```python
from build123d import *

# Parameters (mm, degrees)
SKETCH2_R                        = 25.4
SKETCH2_R_2                      = 14.2875
BOSS_EXTRUDE1_DEPTH              = 38.1
CUT_EXTRUDE1_REACH               = 54.363
SKETCH3_W                        = 25.4
SKETCH3_H                        = 1.5875
CUT_EXTRUDE2_REACH               = 54.363
SKETCH4_R                        = 3.0226
TAP_DRILL_FOR_M4X0_7_TAP1_REACH  = 61.824
TAP_DRILL_FOR_M4X0_7_TAP1_BORE_R = 1.65
CUT_EXTRUDE5_REACH               = 70.392
CUT_EXTRUDE5_END_RADIUS          = 3.0226
SKETCH11_R                       = 1.65
CUT_EXTRUDE6_REACH               = 54.363
TAP_DRILL_FOR_M3X0_5_TAP2_D      = 2.5
TAP_DRILL_FOR_M3X0_5_TAP2_DEPTH  = 4.572
TAP_DRILL_FOR_M3X0_5_TAP2_TIP    = 0.751075774
TAP_DRILL_FOR_M5X0_8_TAP1_REACH  = 55.583
TAP_DRILL_FOR_M5X0_8_TAP1_BORE_R = 2.1
SKETCH15_R                       = 2.665
CUT_EXTRUDE7_DEPTH               = 53.7470617
CUT_EXTRUDE8_REACH               = 59.143
SKETCH19_R                       = 5


with BuildPart() as part:
    # Sketch2 → Boss-Extrude1 (new body)
    with BuildSketch(Plane(origin=(0, 0, 0), x_dir=(1, 0, 0), z_dir=(0, 1, 0))):
        with Locations(Location((0, 0, 0), (0, 0, 90))):
            Circle(SKETCH2_R)
        with Locations(Location((0, 0, 0), (0, 0, 90))):
            Circle(SKETCH2_R_2, mode=Mode.SUBTRACT)
    extrude(amount=BOSS_EXTRUDE1_DEPTH)

    # Sketch3 → Cut-Extrude1 (cut, up to next)
    with BuildSketch(Plane(origin=(0, 38.1, 0), x_dir=(1, 0, 0), z_dir=(0, 1, 0)), mode=Mode.PRIVATE) as cut_extrude1_sk1:
        with Locations((-12.7, 0)):
            Rectangle(SKETCH3_W, SKETCH3_H)
    cut_extrude1_tool1 = extrude(cut_extrude1_sk1.sketch, amount=-CUT_EXTRUDE1_REACH, mode=Mode.PRIVATE) & part.part
    add(cut_extrude1_tool1.solids().sort_by_distance((-12.7, 38.1, 0))[0], mode=Mode.SUBTRACT)

    # Sketch4 → Cut-Extrude2 (cut, up to next)
    with BuildSketch(Plane(origin=(0, 38.1, 0), x_dir=(1, 0, 0), z_dir=(0, 1, 0)), mode=Mode.PRIVATE) as cut_extrude2_sk1:
        with Locations(Location((0, -19.84375, 0), (0, 0, 270))):
            Circle(SKETCH4_R)
    cut_extrude2_tool1 = extrude(cut_extrude2_sk1.sketch, amount=-CUT_EXTRUDE2_REACH, mode=Mode.PRIVATE) & part.part
    cut_extrude2 = cut_extrude2_tool1.solids().sort_by_distance((0, 38.1, 19.84375))[0]
    add(cut_extrude2, mode=Mode.SUBTRACT)

    # Tap Drill for M4x0.7 Tap1 bore (on position points) → Tap Drill for M4x0.7 Tap1 (cut, up to next)
    with BuildSketch(Plane(origin=(-19.826514488, 29.109235595, 0.79375), x_dir=(-1, 0, 0), z_dir=(0, 0, -1)), mode=Mode.PRIVATE) as tap_drill_for_m4x0_7_tap1_sk1:
        Circle(TAP_DRILL_FOR_M4X0_7_TAP1_BORE_R)
    tap_drill_for_m4x0_7_tap1_tool1 = extrude(tap_drill_for_m4x0_7_tap1_sk1.sketch, amount=-TAP_DRILL_FOR_M4X0_7_TAP1_REACH, mode=Mode.PRIVATE) & part.part
    # Tap Drill for M4x0.7 Tap1 bore (on position points) → Tap Drill for M4x0.7 Tap1 (cut, up to next)
    with BuildSketch(Plane(origin=(-19.826514488, 29.109235595, 0.79375), x_dir=(-1, 0, 0), z_dir=(0, 0, -1)), mode=Mode.PRIVATE) as tap_drill_for_m4x0_7_tap1_sk2:
        with Locations((0, -20.205281104)):
            Circle(TAP_DRILL_FOR_M4X0_7_TAP1_BORE_R)
    tap_drill_for_m4x0_7_tap1_tool2 = extrude(tap_drill_for_m4x0_7_tap1_sk2.sketch, amount=-TAP_DRILL_FOR_M4X0_7_TAP1_REACH, mode=Mode.PRIVATE) & part.part
    add(tap_drill_for_m4x0_7_tap1_tool1.solids().sort_by_distance((-19.826514, 29.109236, 0.79375))[0], mode=Mode.SUBTRACT)
    add(tap_drill_for_m4x0_7_tap1_tool2.solids().sort_by_distance((-19.826514, 8.903954, 0.79375))[0], mode=Mode.SUBTRACT)

    # Cut-Extrude5: up to this cylinder (the profile starts outside it)
    cut_extrude5_end = Plane(origin=(0, 19.05, 19.84375), z_dir=(0, 1, 0)) * Cylinder(CUT_EXTRUDE5_END_RADIUS, 147.8292, mode=Mode.PRIVATE)
    # Sketch11 → Cut-Extrude5 (cut, up to the surface)
    with BuildSketch(Plane.XY.offset(25.4), mode=Mode.PRIVATE) as cut_extrude5_sk1:
        with Locations((0.006202687, 19.05)):
            Circle(SKETCH11_R)
    cut_extrude5_tool1 = extrude(cut_extrude5_sk1.sketch, amount=-CUT_EXTRUDE5_REACH, mode=Mode.PRIVATE) - cut_extrude5_end
    cut_extrude5 = cut_extrude5_tool1.solids().sort_by_distance((0.006203, 19.05, 25.4))[0]
    add(cut_extrude5, mode=Mode.SUBTRACT)

    # Mirror1: Cut-Extrude2, Cut-Extrude5 across plane
    add(cut_extrude2.mirror(Plane.XY), mode=Mode.SUBTRACT)
    add(cut_extrude5.mirror(Plane.XY), mode=Mode.SUBTRACT)

    # Sketch12 → Cut-Extrude6 (cut, up to next)
    with BuildSketch(Plane(origin=(0, 38.1, 0), x_dir=(1, 0, 0), z_dir=(0, 1, 0)), mode=Mode.PRIVATE) as cut_extrude6_sk1:
        with BuildLine():
            Line((22.86, 11.071603317), (22.86, -11.071603317))
            ThreePointArc((22.86, -11.071603317), (25.4, 0), (22.86, 11.071603317))
        make_face()
    cut_extrude6_tool1 = extrude(cut_extrude6_sk1.sketch, amount=-CUT_EXTRUDE6_REACH, mode=Mode.PRIVATE) & part.part
    add(cut_extrude6_tool1.solids().sort_by_distance((23.880484, 38.1, 0))[0], mode=Mode.SUBTRACT)

    # Tap Drill for M3x0.5 Tap2
    with Locations(Plane(origin=(22.86, 19.05, 0), x_dir=(0, 0, 1), z_dir=(1, 0, 0))):
        with Locations((0, 0)):
            Hole(TAP_DRILL_FOR_M3X0_5_TAP2_D / 2, depth=TAP_DRILL_FOR_M3X0_5_TAP2_DEPTH)
            with Locations((0, 0, -(TAP_DRILL_FOR_M3X0_5_TAP2_DEPTH + TAP_DRILL_FOR_M3X0_5_TAP2_TIP / 2))):  # 118° drill point
                Cone(0, TAP_DRILL_FOR_M3X0_5_TAP2_D / 2, TAP_DRILL_FOR_M3X0_5_TAP2_TIP, mode=Mode.SUBTRACT)

    # Tap Drill for M5x0.8 Tap1 bore (on position points) → Tap Drill for M5x0.8 Tap1 (cut, up to next)
    with BuildSketch(Plane(origin=(-19.826514488, 19.05, 0.79375), x_dir=(-1, 0, 0), z_dir=(0, 0, -1)), mode=Mode.PRIVATE) as tap_drill_for_m5x0_8_tap1_sk1:
        Circle(TAP_DRILL_FOR_M5X0_8_TAP1_BORE_R)
    tap_drill_for_m5x0_8_tap1_tool1 = extrude(tap_drill_for_m5x0_8_tap1_sk1.sketch, amount=-TAP_DRILL_FOR_M5X0_8_TAP1_REACH, mode=Mode.PRIVATE) & part.part
    add(tap_drill_for_m5x0_8_tap1_tool1.solids().sort_by_distance((-19.826514, 19.05, 0.79375))[0], mode=Mode.SUBTRACT)

    # Sketch15 → Cut-Extrude7 (cut, through all)
    with BuildSketch(Plane(origin=(0, 0, 0.79375), x_dir=(-1, 0, 0), z_dir=(0, 0, -1))):
        with Locations(Location((19.826514488, 19.05, 0), (0, 0, 180))):
            Circle(SKETCH15_R)
    extrude(amount=CUT_EXTRUDE7_DEPTH, mode=Mode.SUBTRACT)

    # Sketch19 → Cut-Extrude8 (cut, up to next)
    with BuildSketch(Plane.XY.offset(-8.79375), mode=Mode.PRIVATE) as cut_extrude8_sk1:
        with Locations((-19.826514488, 19.05)):
            Circle(SKETCH19_R)
    cut_extrude8_tool1 = extrude(cut_extrude8_sk1.sketch, amount=-CUT_EXTRUDE8_REACH, mode=Mode.PRIVATE) & part.part
    add(cut_extrude8_tool1.solids().sort_by_distance((-19.826514, 19.05, -8.79375))[0], mode=Mode.SUBTRACT)


solid = part.part
```
Work out the finished part from the listing and answer in its coordinate system (mm). A direction names the side the tool comes from. Coordinates: 2 decimals unless noted, no trailing zeros. Write each loop counter-clockwise with the first axis right and the second up, starting at its lowest first coordinate (ties: lowest second). Pieces come first, ordered by that corner, then holes. Notation, with made-up numbers: (76, 56.5) - (131, 56.5) arc R25 ccw to (131, 68.5) - close; hole circle Ø1 at (-17, 62.5). An arc over 180 degrees is marked (long way). Answer as a JSON object with one key per item and string values.
Q1. Find section D-D (x = 6). Write down the section's boundary in (y, z), plus the area to 3 significant figures.
Results list:
{"outline": "(0, -24.68) - (38.1, -24.68) - (38.1, -12.97) - (0, -12.97) - close; (0, 12.97) - (38.1, 12.97) - (38.1, 24.68) - (0, 24.68) - close", "area": "893 mm^2"}
Q2. Find section C-C (z = -16). Write down the section's boundary in (x, y).
Results list:
{"outline": "(-19.73, 0) - (19.73, 0) - (19.73, 38.1) - (-19.73, 38.1) - (-19.73, 24.05) arc R5 cw to (-19.73, 14.05) - close"}
Q3. Find section A-A (z = -6.5). Write down the section's boundary in (x, y) (3 decimals), plus the area to 3 significant figures.
Results list:
{"outline": "(-24.554, 0) - (-12.723, 0) - (-12.723, 38.1) - (-24.554, 38.1) - close; (12.723, 0) - (22.86, 0) - (22.86, 38.1) - (12.723, 38.1) - close; hole circle Ø5.33 at (-19.827, 19.05)", "area": "815 mm^2"}
Q4. Given pin 1 Ø4 at (x, y) = (0.01, 19.05) entering from -Z; pin 2 Ø4.5 at (x, y) = (-19.83, 8.9) entering from +Z; pin 3 Ø1.5 at (x, y) = (-13.5, 4) entering from -Z; pin 4 Ø6 at (y, z) = (16, 6) entering from -X, each flat-ended and moving along its own axis, determine where each tip first touches the part or whether it passes through.
Results list:
{"pin 1": "stops at z = -25.4", "pin 2": "stops at z = 18.33", "pin 3": "stops at z = -21.97", "pin 4": "stops at x = -25.22"}
Q5. For a pull along Z with two mould halves and no side action, classify faces 6 (the cylindrical face through (-4.829, 18.783, -24.937)), 7 (the cylindrical face through (1.58, 19.55, 23.91)), 8 (the flat face through (-17, 19, 0.794)) as pulls with the +Z half, pulls with the -Z half, needs draft (parallel to the pull), parting line crosses it, or undercut.
Results list:
{"face 6": "pulls with the -Z half", "face 7": "needs draft", "face 8": "undercut"}
Q6. Find section B-B (x = -12.5). Write down the section's boundary in (y, z).
Results list:
{"outline": "(0, -22.11) - (38.1, -22.11) - (38.1, -6.92) - (0, -6.92) - close; (0, 6.92) - (38.1, 6.92) - (38.1, 22.11) - (0, 22.11) - close"}
Q7. Which of the six approach directions +Z, -Z, +X, -X, +Y, -Y give full straight-line access (tool end or side, diameter ignored) to faces 1 (the cylindrical face through (1.58, 19.55, -23.91)), 2 (the cylindrical face through (-18.18, 8.98, 9.15)), 3 (the flat face through (9, 38.1, 12)), 4 (the flat face through (-16, 19, -0.794)), 5 (the cylindrical face through (20.542, 17.996, -0.672))?
Results list:
{"face 1": "-Z", "face 2": "+Z", "face 3": "+Z, -Z, +X, -X, +Y", "face 4": "-X, +Y, -Y", "face 5": "+X"}
Q8. Consider L1, parallel to Y at x = -20, z = 1; L2, parallel to X at y = 20, z = -7.5; L3, parallel to Z at x = -21, y = 32.5. Determine where each line is inside the solid, lowest interval first. Write a range as from..to.
Results list:
{"L1": "y = 0..7.26, 10.54..16.96, 21.14..27.47, 30.75..38.1", "L2": "x = -24.27..-22.32, -17.34..-12.16, 12.16..22.86", "L3": "z = -14.29..-0.79, 0.79..14.29"}
